Read the model definition and answer for the solid it produces. Units are mm, in the model's axes. A direction names the side the tool comes from. Give positions to 0.01 mm unless a question says otherwise; leave off trailing zeros. Order: outer loops, then holes, each group sorted by start corner. A loop starts at its lowest first (then second) coordinate and runs counter-clockwise, first axis right, second up.
```python
from build123d import *

# Parameters (mm, degrees)
SKETCH1_W           = 42
SKETCH1_H           = 65.5
BOSS_EXTRUDE1_DEPTH = 9
CUT_EXTRUDE2_DEPTH  = 4.5
SKETCH3_R           = 1.75
CUT_EXTRUDE5_DEPTH  = 78.939078773
SKETCH5_R           = 3
CUT_EXTRUDE6_DEPTH  = 3.25
FILLET1_R           = 4
SKETCH6_R           = 1.75
CUT_EXTRUDE7_DEPTH  = 79.327836687
SKETCH7_R           = 3
CUT_EXTRUDE8_DEPTH  = 3


with BuildPart() as part:
    # Sketch1 → Boss-Extrude1 (new body)
    with BuildSketch(Plane.XY):
        with Locations((21, 32.75)):
            Rectangle(SKETCH1_W, SKETCH1_H)
    extrude(amount=BOSS_EXTRUDE1_DEPTH)

    # Sketch2 → Cut-Extrude2 (cut)
    with BuildSketch(Plane(origin=(0, 0, 0), x_dir=(-1, 0, 0), z_dir=(0, 0, -1))):
        with BuildLine():
            Line((-25.5, 21.25), (-25.5, 35.084635496))
            ThreePointArc((-25.5, 35.084635496), (-25.998538124, 38.202683318), (-27.444444444, 41.009837998))
            ThreePointArc((-27.444444444, 41.009837998), (-21, 53.75), (-14.555555556, 41.009837998))
            ThreePointArc((-14.555555556, 41.009837998), (-16.001461876, 38.202683318), (-16.5, 35.084635496))
            Line((-16.5, 35.084635496), (-16.5, 21.25))
            ThreePointArc((-16.5, 21.25), (-21, 16.75), (-25.5, 21.25))
        make_face()
    extrude(amount=-CUT_EXTRUDE2_DEPTH, mode=Mode.SUBTRACT)

    # Sketch3 → Cut-Extrude5 (cut, through all)
    with BuildSketch(Plane(origin=(0, 0, 4.5), x_dir=(-1, 0, 0), z_dir=(0, 0, -1))):
        with Locations((-21, 21.25)):
            Circle(SKETCH3_R)
        with Locations((-21, 45.75)):
            Circle(SKETCH3_R)
    extrude(amount=-CUT_EXTRUDE5_DEPTH, mode=Mode.SUBTRACT)

    # Sketch5 → Cut-Extrude6 (cut)
    with BuildSketch(Plane.XY.offset(9)):
        with Locations((21, 21.25)):
            Circle(SKETCH5_R)
        with Locations((21, 45.75)):
            Circle(SKETCH5_R)
    extrude(amount=-CUT_EXTRUDE6_DEPTH, mode=Mode.SUBTRACT)

    # Fillet1
    fillet1_edges = [part.edges().sort_by_distance(p)[0] for p in [
        (21, 65.5, 0),
        (21, 0, 0),
    ]]
    fillet(fillet1_edges, radius=FILLET1_R)

    # Sketch6 → Cut-Extrude7 (cut, through all)
    with BuildSketch(Plane(origin=(0, 0, 0), x_dir=(-1, 0, 0), z_dir=(0, 0, -1))):
        with BuildLine():
            Line((-5.75, 4), (-2.25, 4))
            ThreePointArc((-2.25, 4), (-4, 5.75), (-5.75, 4))
        make_face()
        with BuildLine():
            ThreePointArc((-5.75, 4), (-4, 2.25), (-2.25, 4))
            Line((-2.25, 4), (-5.75, 4))
        make_face()
        with BuildLine():
            ThreePointArc((-39.75, 4), (-38, 2.25), (-36.25, 4))
            Line((-36.25, 4), (-39.75, 4))
        make_face()
        with BuildLine():
            Line((-39.75, 4), (-36.25, 4))
            ThreePointArc((-36.25, 4), (-38, 5.75), (-39.75, 4))
        make_face()
        with Locations((-38, 61.5)):
            Circle(SKETCH6_R)
        with Locations((-4, 61.5)):
            Circle(SKETCH6_R)
    extrude(amount=-CUT_EXTRUDE7_DEPTH, mode=Mode.SUBTRACT)

    # Sketch7 → Cut-Extrude8 (cut)
    with BuildSketch(Plane(origin=(0, 0, 0), x_dir=(-1, 0, 0), z_dir=(0, 0, -1))):
        with Locations((-38, 61.5)):
            Circle(SKETCH7_R)
        with Locations((-4, 61.5)):
            Circle(SKETCH7_R)
        with Locations((-4, 4)):
            Circle(SKETCH7_R)
        with Locations((-38, 4)):
            Circle(SKETCH7_R)
    extrude(amount=-CUT_EXTRUDE8_DEPTH, mode=Mode.SUBTRACT)


solid = part.part
```
1) A tool of negligible diameter and unlimited length cuts with its end or side. For faces 1 (the face through (21, 19, 5.75)), 2 (the face through (22.29, 22.43, 5.12)), 3 (the face through (38, 7, 1)), from which of +Z, -Z, +X, -X, +Y, -Y can it reach the whole face along a straight path? Write none if from no direction.
Final values:
face 1: +Z
face 2: +Z, -Z
face 3: -Z
2) For a pull along X with two mould halves and no side action, classify faces 4 (the face through (21, 0, 6)), 5 (the face through (0, 32, 4)), 6 (the face through (38.65, 58.57, 1.48)) as released by +X, released by -X, zero draft, split by the parting line, or undercut.
Final values:
face 4: zero draft
face 5: released by -X
face 6: undercut
3) The part is cut by section C-C on x = 5. Determine the outline of the cut face in (y, z).
Final values:
outline: (0, 4) arc R4 ccw to (1.17, 1.17) - (1.17, 3) - (2.56, 3) - (2.56, 9) - (0, 9) - close; (5.44, 3) - (6.83, 3) - (6.83, 0) - (58.67, 0) - (58.67, 3) - (60.06, 3) - (60.06, 9) - (5.44, 9) - close; (62.94, 3) - (64.33, 3) - (64.33, 1.17) arc R4 ccw to (65.5, 4) - (65.5, 9) - (62.94, 9) - close
4) The part is cut by section D-D on x = 38. Determine the outline of the cut face in (y, z).
Final values:
outline: (0, 4) arc R4 ccw to (1, 1.35) - (1, 3) - (2.25, 3) - (2.25, 9) - (0, 9) - close; (5.75, 3) - (7, 3) - (7, 0) - (58.5, 0) - (58.5, 3) - (59.75, 3) - (59.75, 9) - (5.75, 9) - close; (63.25, 3) - (64.5, 3) - (64.5, 1.35) arc R4 ccw to (65.5, 4) - (65.5, 9) - (63.25, 9) - close
5) The part is cut by section B-B on z = 8.25. Determine the outline of the cut face in (x, y), and give its area (3 significant figures).
Final values:
outline: (0, 0) - (42, 0) - (42, 65.5) - (0, 65.5) - close; hole circle Ø3.5 at (4, 4); hole circle Ø3.5 at (4, 61.5); hole circle Ø6 at (21, 21.25); hole circle Ø6 at (21, 45.75); hole circle Ø3.5 at (38, 4); hole circle Ø3.5 at (38, 61.5)
area: 2,660 mm2
6) The part is cut by section A-A on y = 45.75. Determine the outline of the cut face in (x, z), and give its area (3 significant figures).
Final values:
outline: (0, 0) - (13, 0) - (13, 4.5) - (19.25, 4.5) - (19.25, 5.75) - (18, 5.75) - (18, 9) - (0, 9) - close; (22.75, 4.5) - (29, 4.5) - (29, 0) - (42, 0) - (42, 9) - (24, 9) - (24, 5.75) - (22.75, 5.75) - close
area: 282 mm2
7) Consider L1, parallel to Y at x = 38, z = 4.7; L2, parallel to X at y = 4, z = 1.15; L3, parallel to X at y = 29.5, z = 1.5. Determine where each line is inside the solid, lowest interval first.
Final values:
L1: y = 0 to 2.25, 5.75 to 59.75, 63.25 to 65.5
L2: x = 0 to 1, 7 to 35, 41 to 42
L3: x = 0 to 16.5, 25.5 to 42
8) Given pin 1 (3 mm diameter, centred on x = 37.5, y = 4.5, fed in from -Z); pin 2 (4 mm diameter, centred on x = 21, y = 21.25, fed in from +Z); pin 3 (4 mm diameter, centred on x = 21, y = 45.75, fed in from -Z), each flat-ended and moving along its own axis, determine where each tip first touches the part or whether it passes through.
Final values:
pin 1: stops at z = 3
pin 2: stops at z = 5.75
pin 3: stops at z = 4.5
